Could you check a few things on this model? Use its own coordinates, in mm. Face numbers are marked on the shaded views. A direction names the side the tool comes from. Round coordinates to 2 decimals unless told otherwise and drop trailing zeros. Write each loop counter-clockwise with the first axis right and the second up, starting at its lowest first coordinate (ties: lowest second). Pieces come first, ordered by that corner, then holes. Notation, with made-up numbers: (50, 42.25) - (102, 42.25) arc R19 ccw to (102, 54.25) - close; hole circle Ø10 at (67, 35). An arc over 180 degrees is marked (long way). Write each question's results on one line, items separated by ' | '. Start each with the question number.
(1) Please list where these lines run through material, in increasing order: line 1 (Z direction, x = -1.6, y = -0.5); line 2 (Y direction, x = 1.25, z = -4); line 3 (X direction, y = 0.85, z = -21.75). Write a range as [from, to].
(2) On a 3-axis mill with a long thin cutter (end or side, diameter ignored), from which of +Z, -Z, +X, -X, +Y, -Y can I reach the whole of each face in a straight line? I mean the marked faces 1, 2 and 3. Say none if no direction works.
(3) For P1, Ø2, axis at y = -1, z = -14.5, coming from the -X side; P2, Ø2, axis at y = -1, z = -14, coming from the +X side; P3, Ø1.5, axis at x = -2, z = -20.5, coming from the +Y side, each with a flat end and sliding along its axis, tell me the tip position at first contact or that it passes through.
(4) Imagine slicing it at C-C on z = -16. Write out the boundary of the cut face in (x, y), then the cut area to 3 significant figures.
(5) Imagine slicing it at B-B on z = -7.75. Write out the boundary of the cut face in (x, y), then the cut area to 3 significant figures.
(6) Imagine slicing it at A-A on x = 0. Write out the boundary of the cut face in (y, z), then the cut area to 3 significant figures.
```python
from build123d import *

# Parameters (mm, degrees)
SKETCH015_R  = 1.75
SKETCH016_R  = 2.5
SKETCH017_R  = 1.5
PAD007_DEPTH = 20
SKETCH014_R  = 1.75
PAD008_DEPTH = 3


with BuildPart() as part:
    # Sketch015 → AdditiveLoft001 section 0
    with BuildSketch(Plane.XY.offset(-5)):
        Circle(SKETCH015_R)
    # Sketch016 → AdditiveLoft001 section 1
    with BuildSketch(Plane.XY.offset(-9)):
        Circle(SKETCH016_R)
    loft()

    # Sketch017 → Pad007 (new body)
    with BuildSketch(Plane.XY.offset(-9)):
        Circle(SKETCH017_R)
    extrude(amount=-PAD007_DEPTH)

    # Sketch014 → Pad008 (join)
    with BuildSketch(Plane.XY.offset(-5)):
        Circle(SKETCH014_R)
    extrude(amount=PAD008_DEPTH)


solid = part.part
```
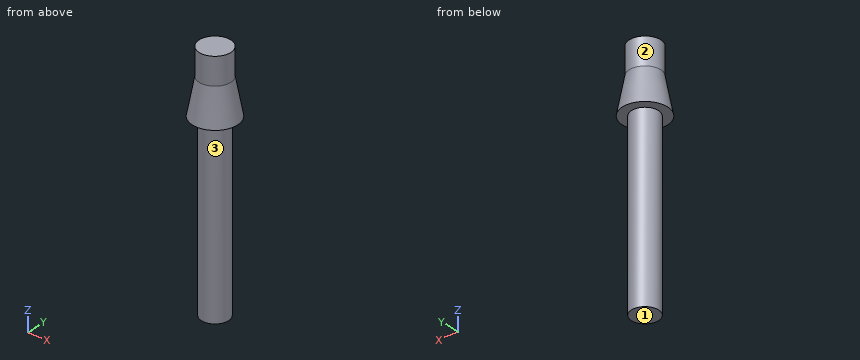
Response:
1) line 1: [-9, -2] | line 2: [-1.22, 1.22] | line 3: [-1.24, 1.24]
2) face 1: -Z, +X, -X, +Y, -Y | face 2: +Z | face 3: -Z
3) P1: x = -1.5 | P2: x = 1.5 | P3: y = 0.83
4) outline: circle Ø3 at (0, 0) | area: 7.07 mm²
5) outline: circle Ø4.53 at (0, 0) | area: 16.1 mm²
6) outline: (-2.5, -9) - (-1.5, -9) - (-1.5, -29) - (1.5, -29) - (1.5, -9) - (2.5, -9) - (1.75, -5) - (1.75, -2) - (-1.75, -2) - (-1.75, -5) - close | area: 87.5 mm²
